Part model, mm, in its own coordinate system. Face numbers are marked on the shaded views. A direction names the side the tool comes from. Round coordinates to 2 decimals unless told otherwise and drop trailing zeros. Order: outer loops, then holes, each group sorted by start corner. A loop starts at its lowest first (then second) coordinate and runs counter-clockwise, first axis right, second up. Notation, with made-up numbers: (67, 60) - (112, 60) arc R18 ccw to (112, 85) - close; hole circle Ø1 at (65.5, 75.25). An arc over 180 degrees is marked (long way). Return JSON: item names as keys, results as strings. Group by question number.
Item 1: Two-plate mould, pull along Z, no slides. Class the marked faces 3, 4 and 5: released by +Z, released by -Z, zero draft, split by the parting line, or undercut.
Item 2: Drop a flat-ended pin along its axis: pin 1 (2 mm diameter, centred on x = 1.5, y = 4, fed in from +Z). Give the stop position or say it passes through.
Item 3: Saw through at A-A on z = 0. List the corners of the cut face in (x, y) (3 decimals).
Item 4: Probe probe 1 along Y at (x, z) = (0.5, 1.65); probe 2 along Z at (x, y) = (0, 4.75); probe 3 along Z at (x, y) = (-0.65, 0.5). List the from-to ranges inside material, lowest first.
Item 5: Tool access for the marked faces 1 and 2: list every direction of +Z, -Z, +X, -X, +Y, -Y with a clear straight run to the whole face (end or side of a thin tool).
Item 6: Saw through at D-D on y = 3.75. List the corners of the cut face in (x, z) (3 decimals), and give its area (3 significant figures).
Item 7: Saw through at B-B on x = 0. List the corners of the cut face in (y, z) (3 decimals).
Item 8: Saw through at C-C on y = 1.25. List the corners of the cut face in (x, z).
```python
from build123d import *

# Parameters (mm, degrees)
SKETCH1_R           = 2.15
BOSS_EXTRUDE1_DEPTH = 6.6
SKETCH2_R           = 1
CUT_EXTRUDE1_DEPTH  = 7.6
SKETCH3_R           = 2.15
SKETCH3_R_2         = 1.125
CUT_EXTRUDE2_DEPTH  = 1.25


with BuildPart() as part:
    # Sketch1 → Boss-Extrude1 (new body)
    with BuildSketch(Plane(origin=(0, 0, 0), x_dir=(1, 0, 0), z_dir=(0, 1, 0))):
        Circle(SKETCH1_R)
    extrude(amount=BOSS_EXTRUDE1_DEPTH)

    # Sketch2 → Cut-Extrude1 (cut, through all)
    with BuildSketch(Plane.XZ):
        Circle(SKETCH2_R)
    extrude(amount=-CUT_EXTRUDE1_DEPTH, mode=Mode.SUBTRACT)

    # Sketch3 → Cut-Extrude2 (cut)
    with BuildSketch(Plane(origin=(0, 4.25, 0), x_dir=(-1, 0, 0), z_dir=(0, -1, 0))):
        Circle(SKETCH3_R)
        Circle(SKETCH3_R_2, mode=Mode.SUBTRACT)
    extrude(amount=CUT_EXTRUDE2_DEPTH, mode=Mode.SUBTRACT)


solid = part.part
```
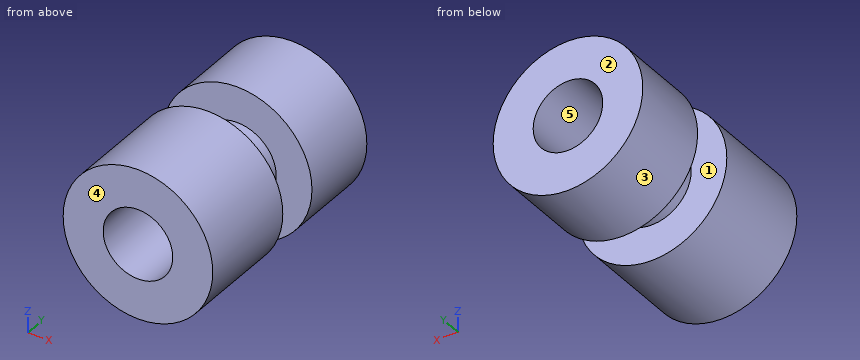
Filled in:
{
 "1": {"face 3": "split by the parting line", "face 4": "zero draft", "face 5": "undercut"},
 "2": {"pin 1": "stops at z = 2.08"},
 "3": {"outline": "(-2.15, 0) - (-1, 0) - (-1, 6.6) - (-2.15, 6.6) - (-2.15, 4.25) - (-1.125, 4.25) - (-1.125, 3) - (-2.15, 3) - close; (1, 0) - (2.15, 0) - (2.15, 3) - (1.125, 3) - (1.125, 4.25) - (2.15, 4.25) - (2.15, 6.6) - (1, 6.6) - close"},
 "4": {"probe 1": "y = 0 to 3, 4.25 to 6.6", "probe 2": "z = -2.15 to -1, 1 to 2.15", "probe 3": "z = -2.05 to -0.76, 0.76 to 2.05"},
 "5": {"face 1": "none", "face 2": "+Z, -Z, +X, -X, +Y"},
 "6": {"outline": "circle Ø2.25 at (0, 0); hole circle Ø2 at (0, 0)", "area": "0.834 mm^2"},
 "7": {"outline": "(0, -2.15) - (3, -2.15) - (3, -1.125) - (4.25, -1.125) - (4.25, -2.15) - (6.6, -2.15) - (6.6, -1) - (0, -1) - close; (0, 1) - (6.6, 1) - (6.6, 2.15) - (4.25, 2.15) - (4.25, 1.125) - (3, 1.125) - (3, 2.15) - (0, 2.15) - close"},
 "8": {"outline": "circle Ø4.3 at (0, 0); hole circle Ø2 at (0, 0)"}
}
